Here's the drawing with two shaded views (mm, measured from the low corner). I have some questions. A direction names the side the tool comes from. Round coordinates to 2 decimals unless told otherwise and drop trailing zeros. Loops run counter-clockwise (first coordinate to the right, second up) from the corner with the lowest first, then second, coordinate; pieces in that order, holes last.
(1) I want a section at D-D on x = 6. Write out the boundary of the cut face in (y, z) (3 decimals), plus the area to 3 significant figures.
(2) I want a section at A-A on z = 1.9. Write out the boundary of the cut face in (x, y).
(3) I want a section at B-B on y = 3.75. Write out the boundary of the cut face in (x, z).
(4) Thinking about a two-plate mould opening in X: for the marked faces 1, 2 and 3, which applies, released by +X, released by -X, zero draft, split by the parting line, or undercut?
(5) Will these pins go through, and if not, where does the flat tip stop? pin 1 Ø1.2 at (y, z) = (3, 0.5) entering from +X; pin 2 Ø1.5 at (x, z) = (2, 2.5) entering from +Y; pin 3 Ø2 at (y, z) = (1.5, 0.5) entering from +X.
(6) Which directions (+Z, -Z, +X, -X, +Y, -Y) give clear straight access to the entire face, cutting with the end or side of a thin tool? Please do the marked faces 4 and 5.
(7) If I drill on line 1 along Y through (x, z) = (3.75, 2.85); line 2 along Y through (x, z) = (2, 0.35); line 3 along Z through (x, y) = (5.25, 6.25), over which ranges is the centre line in solid material (lowest first)?
(8) I want a section at C-C on x = 2.5. Write out the boundary of the cut face in (y, z), plus the area to 3 significant figures.
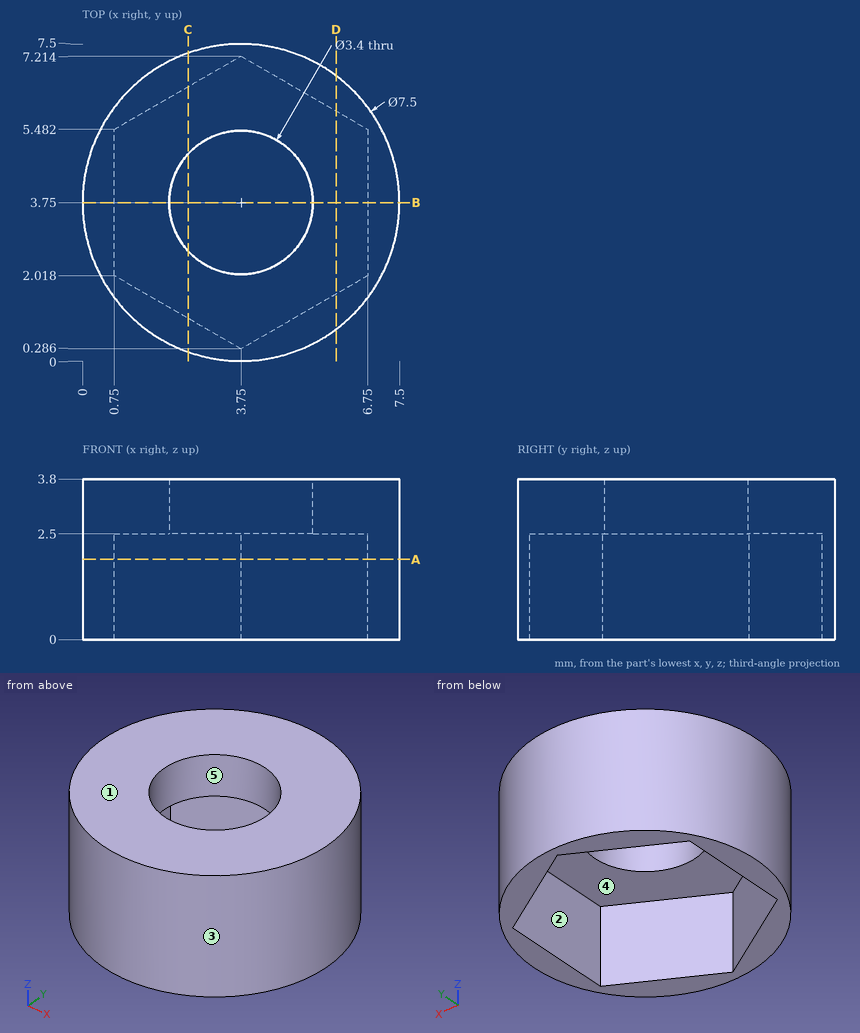
Filled sheet:
1. outline: (0.75, 0) - (1.585, 0) - (1.585, 2.5) - (5.915, 2.5) - (5.915, 0) - (6.75, 0) - (6.75, 3.8) - (0.75, 3.8) - close
1. area: 12.0 mm2
2. outline: circle Ø7.5 at (3.75, 3.75); hole (0.75, 2.02) - (3.75, 0.29) - (6.75, 2.02) - (6.75, 5.48) - (3.75, 7.21) - (0.75, 5.48) - close
3. outline: (0, 0) - (0.75, 0) - (0.75, 2.5) - (2.05, 2.5) - (2.05, 3.8) - (0, 3.8) - close; (5.45, 2.5) - (6.75, 2.5) - (6.75, 0) - (7.5, 0) - (7.5, 3.8) - (5.45, 3.8) - close
4. face 1: zero draft
4. face 2: undercut
4. face 3: split by the parting line
5. pin 1: stops at x = 7.5
5. pin 2: stops at y = 7.36
5. pin 3: stops at x = 7.29
6. face 4: -Z
6. face 5: +Z, -Z
7. line 1: y = 0 to 2.05, 5.45 to 7.5
7. line 2: y = 0.43 to 1.3, 6.2 to 7.07
7. line 3: z = 2.5 to 3.8
8. outline: (0.21, 0) - (1.01, 0) - (1.01, 2.5) - (2.6, 2.5) - (2.6, 3.8) - (0.21, 3.8) - close; (4.9, 2.5) - (6.49, 2.5) - (6.49, 0) - (7.29, 0) - (7.29, 3.8) - (4.9, 3.8) - close
8. area: 10.2 mm2
